```python
from build123d import *

# Parameters (mm, degrees)
F0_W     = 76.410934
F0_H     = 127
F1_DEPTH = 2.54
F2_R     = 5.08
F3_W     = 20.763844
F3_H     = 58.415605
F4_DEPTH = 13.97


with BuildPart() as f1:
    # F0 (on Front) → F1 (new body)
    with BuildSketch(Plane.XZ):
        with Locations((-2.076384, 0.516346)):
            Rectangle(F0_W, F0_H)
    extrude(amount=F1_DEPTH)

    # F2
    f2_edges = [f1.edges().sort_by_distance(p)[0] for p in [
        (-40.281851, -1.27, 64.016346),
        (36.129083, -1.27, 64.016346),
        (36.129083, -1.27, -62.983654),
        (-40.281851, -1.27, -62.983654),
    ]]
    fillet(f2_edges, radius=F2_R)

    # F3 (on Front) → F4 (join)
    with BuildSketch(Plane.XZ):
        with Locations((-0.553702, 1.937959)):
            Rectangle(F3_W, F3_H)
    extrude(amount=F4_DEPTH)


solid = f1.part
```
Input: part model. Units: mm. Frame: model coordinates. A direction names the side the tool comes from. Coordinates: 2 decimals unless noted, no trailing zeros. Order: outer loops, then holes, each group sorted by start corner. A loop starts at its lowest first (then second) coordinate and runs counter-clockwise, first axis right, second up. Notation, with made-up numbers: (-33, 53.5) - (15, 53.5) arc R19 cw to (15, 90.5) - close; hole circle Ø7 at (-34.75, -39.5). An arc over 180 degrees is marked (long way). Return JSON: item names as keys, results as strings.
Q1. Cut plane B-B (x = 3). Return loops of the section in (y, z), then the cut area to 3 significant figures.
The answers:
{"outline": "(-13.97, -27.27) - (-2.54, -27.27) - (-2.54, -62.98) - (0, -62.98) - (0, 64.02) - (-2.54, 64.02) - (-2.54, 31.15) - (-13.97, 31.15) - close", "area": "990 mm2"}
Q2. Access query for faces 4 (the cylindrical face through (34.601, -1.288, -61.535)), 5 (the flat face through (-1, -8, 31.146)), 6 (the flat face through (-1, -8, -27.27)), 7 (the flat face through (-10.936, -8, 2)), 8 (the flat face through (-40.282, -1, 0)). Directions: +Z, -Z, +X, -X, +Y, -Y. A direction counts if a zero-diameter tool reaches every point of the face in a straight line with its end or side. Return the directions, or none.
The answers:
{"face 4": "-Z, +X, +Y, -Y", "face 5": "+Z, +X, -X, -Y", "face 6": "-Z, +X, -X, -Y", "face 7": "+Z, -Z, -X, -Y", "face 8": "+Z, -Z, -X, +Y, -Y"}
Q3. Cut plane A-A (z = 28). Return loops of the section in (x, y), then the cut area to 3 significant figures.
The answers:
{"outline": "(-40.28, -2.54) - (-10.94, -2.54) - (-10.94, -13.97) - (9.83, -13.97) - (9.83, -2.54) - (36.13, -2.54) - (36.13, 0) - (-40.28, 0) - close", "area": "431 mm2"}
Q4. First-contact query: pin 1 (8 mm diameter, centred on x = -11.5, y = -11, fed in from +Z); pin 2 (3.5 mm diameter, centred on y = -8, z = 2.5, fed in from -X); pin 3 (5.5 mm diameter, centred on y = -10.5, z = -3.5, fed in from +X). Flat tips, straight axial feed; report the tip coordinate or a pass-through.
The answers:
{"pin 1": "stops at z = 31.15", "pin 2": "stops at x = -10.94", "pin 3": "stops at x = 9.83"}
Q5. Ray query, probe 1 along Y at (x, z) = (13.5, -4.5); probe 2 along Z at (x, y) = (7.5, -7.75); probe 3 along X at (y, z) = (-6.75, -19.5). Return the intervals inside material, ascending.
The answers:
{"probe 1": "y = -2.54 to 0", "probe 2": "z = -27.27 to 31.15", "probe 3": "x = -10.94 to 9.83"}
Q6. Cut plane C-C (y = -12.5). Return loops of the section in (x, z).
The answers:
{"outline": "(-10.94, -27.27) - (9.83, -27.27) - (9.83, 31.15) - (-10.94, 31.15) - close"}
Q7. Draft query along Y for faces 1 (the flat face through (-3, 0, 1)), 2 (the flat face through (-1, -13.97, 2)), 3 (the flat face through (9.828, -8, 2)). Return one class per face: +Y half, -Y half, draft (parallel to the pull), parting line (faces both ways), or undercut.
The answers:
{"face 1": "+Y half", "face 2": "-Y half", "face 3": "draft"}
Q8. Cut plane D-D (z = 44.5). Return loops of the section in (x, y).
The answers:
{"outline": "(-40.28, -2.54) - (36.13, -2.54) - (36.13, 0) - (-40.28, 0) - close"}
